The listing builds one solid part. Answer for the finished solid, in the listing's coordinates (mm). A direction names the side the tool comes from. Round coordinates to 2 decimals unless told otherwise and drop trailing zeros. Order: outer loops, then holes, each group sorted by start corner. A loop starts at its lowest first (then second) coordinate and runs counter-clockwise, first axis right, second up. Notation, with made-up numbers: M 35,19 L 54,19 A22 ccw 54,33 Z; hole C -19.75,83 d10. An arc over 180 degrees is marked long. Put each result on its own line as item: value. Start each with the question number.
1. Each of these flat-tipped pins is pushed along its axis until it touches: pin 1 Ø3.5 at (x, y) = (74.8, 35) entering from -Z; pin 2 Ø2 at (y, z) = (50, 3) entering from -X; pin 3 Ø2 at (y, z) = (6.5, 0.5) entering from +X; pin 4 Ø2 at (x, z) = (-79.5, 2) entering from +Y. Where does it stop, or does it pass through?
2. Consider line 1 (Y direction, x = -15.5, z = 1.1); line 2 (X direction, y = -45.5, z = 2.75); line 3 (X direction, y = -6, z = 1.25). Determine where each line is inside the solid, lowest interval first.
3. The mould has two halves that part along X. Classify faces 1 (the face through (77.8, 50, 2)), 2 (the face through (-80, 20, 2)), 3 (the face through (13.262, 13.632, 2.028)): +X half, -X half, draft (parallel to the pull), parting line (faces both ways), or undercut.
4. The part is cut by section B-B (z = 1). Count the separate pieces of the cut face and the enclosed holes in it, then the cut area to 3 significant figures.
5. The part is cut by section A-A (y = 6). Give the vertices of the cut face in (x, z).
6. Which of the six approach directions +Z, -Z, +X, -X, +Y, -Y give full straight-line access (tool end or side, diameter ignored) to faces 4 (the face through (-77.8, 50, 2)), 5 (the face through (80, 0, 2)), 6 (the face through (-80, 0, 2))?
from build123d import *

# Parameters (mm, degrees)
EXTRUDE_1_DEPTH     = 4
FILLET_1_R          = 3
SKETCH_2_R          = 1.5
SKETCH_2_R_2        = 2
CUT_EXTRUDE_1_DEPTH = 4


with BuildPart() as part:
    # Sketch 1 → Extrude 1 (new body)
    with BuildSketch(Plane.XY):
        with BuildLine():
            Line((77.8, 60), (-77.8, 60))
            Line((-77.8, 60), (-77.8, 43))
            ThreePointArc((-77.8, 43), (-76.3, 41.5), (-77.8, 40))
            Line((-77.8, 40), (-81.8, 40))
            Line((-81.8, 40), (-81.8, 20))
            Line((-81.8, 20), (-77.8, 20))
            ThreePointArc((-77.8, 20), (-76.3, 18.5), (-77.8, 17))
            Line((-77.8, 17), (-77.8, 3))
            ThreePointArc((-77.8, 3), (-76.3, 1.5), (-77.8, 0))
            Line((-77.8, 0), (-81.8, 0))
            Line((-81.8, 0), (-81.8, -20))
            Line((-81.8, -20), (-77.8, -20))
            ThreePointArc((-77.8, -20), (-76.3, -21.5), (-77.8, -23))
            Line((-77.8, -23), (-77.8, -37))
            ThreePointArc((-77.8, -37), (-76.3, -38.5), (-77.8, -40))
            Line((-77.8, -40), (-81.8, -40))
            Line((-81.8, -40), (-81.8, -60))
            Line((-81.8, -60), (81.8, -60))
            Line((81.8, -60), (81.8, -40))
            Line((81.8, -40), (77.8, -40))
            ThreePointArc((77.8, -40), (76.3, -38.5), (77.8, -37))
            Line((77.8, -37), (77.8, -23))
            ThreePointArc((77.8, -23), (76.3, -21.5), (77.8, -20))
            Line((77.8, -20), (81.8, -20))
            Line((81.8, -20), (81.8, 0))
            Line((81.8, 0), (77.8, 0))
            ThreePointArc((77.8, 0), (76.3, 1.5), (77.8, 3))
            Line((77.8, 3), (77.8, 17))
            ThreePointArc((77.8, 17), (76.3, 18.5), (77.8, 20))
            Line((77.8, 20), (81.8, 20))
            Line((81.8, 20), (81.8, 40))
            Line((81.8, 40), (77.8, 40))
            ThreePointArc((77.8, 40), (76.3, 41.5), (77.8, 43))
            Line((77.8, 43), (77.8, 60))
        make_face()
    extrude(amount=EXTRUDE_1_DEPTH)

    # Fillet 1
    fillet_1_edges = [part.edges().sort_by_distance(p)[0] for p in [
        (81.8, -60, 2),
        (-81.8, -60, 2),
        (-77.8, 60, 2),
        (77.8, 60, 2),
    ]]
    fillet(fillet_1_edges, radius=FILLET_1_R)

    # Sketch 2 → Cut-Extrude 1 (cut)
    with BuildSketch(Plane.XY.offset(4)):
        with Locations((-74.8, 55)):
            Circle(SKETCH_2_R)
        with Locations((-74.8, 35)):
            Circle(SKETCH_2_R)
        with Locations((-74.8, 15)):
            Circle(SKETCH_2_R)
        with Locations((-74.8, -5)):
            Circle(SKETCH_2_R)
        with Locations((-74.8, -25)):
            Circle(SKETCH_2_R)
        with Locations((-74.8, -45)):
            Circle(SKETCH_2_R)
        with Locations(Location((74.8, -45, 0), (0, 0, 180))):
            Circle(SKETCH_2_R)
        with Locations(Location((74.8, -25, 0), (0, 0, 180))):
            Circle(SKETCH_2_R)
        with Locations(Location((74.8, -5, 0), (0, 0, 180))):
            Circle(SKETCH_2_R)
        with Locations(Location((74.8, 15, 0), (0, 0, 180))):
            Circle(SKETCH_2_R)
        with Locations(Location((74.8, 35, 0), (0, 0, 180))):
            Circle(SKETCH_2_R)
        with Locations(Location((74.8, 55, 0), (0, 0, 180))):
            Circle(SKETCH_2_R)
        with Locations((-14.849242405, 14.849242405)):
            Circle(SKETCH_2_R_2)
        with Locations((14.849242405, 14.849242405)):
            Circle(SKETCH_2_R_2)
        with Locations((14.849242405, -14.849242405)):
            Circle(SKETCH_2_R_2)
        with Locations((-14.849242405, -14.849242405)):
            Circle(SKETCH_2_R_2)
    extrude(amount=-CUT_EXTRUDE_1_DEPTH, mode=Mode.SUBTRACT)


solid = part.part
Resolved:
1. pin 1: z = 0
1. pin 2: x = -77.8
1. pin 3: x = 77.8
1. pin 4: y = 40
2. line 1: -60 to -16.74, -12.96 to 12.96, 16.74 to 60
2. line 2: -81.8 to -76.21, -73.39 to 73.39, 76.21 to 81.8
2. line 3: -81.8 to -75.92, -73.68 to 73.68, 75.92 to 81.8
3. face 1: +X half
3. face 2: draft
3. face 3: undercut
4. separate pieces: 1
4. enclosed holes: 16
4. area: 19,000 mm2
5. outline: M -77.8,0 L 77.8,0 L 77.8,4 L -77.8,4 Z
6. face 4: +Z, -Z, -X, +Y
6. face 5: +Z, -Z, +X
6. face 6: +Z, -Z, -X
